Solid Edge part; units mm, degrees
sketch "Sketch1" plane through (0, 0, 0) normal (0, -1, 0) x (1, 0, 0)
  line L0 (25, 129.6172) -> (42.2199, 3)
  line L1 (50, 3) -> (42.2199, 3)
  line L2 (50, 0) -> (50, 3)
  line L3 (50, 0) -> (70, 0)
  line L4 (70, 0) -> (70, 20)
  line L5 (70, 20) -> (50, 20)
  line L6 (33, 145) -> (50, 20)
  line L7 (35, 145) -> (33, 145)
  line L8 (35, 185) -> (35, 145)
  line L9 (25, 185) -> (35, 185)
  line L10 (25, 185) -> (25, 129.6172)
  dimension "D1" = 70
  dimension "D2" = 50
  dimension "D3" = 70
  dimension "D4" = 35
  dimension "D5" = 35
revolve "RevolvedProtrusion1" add sketch "Sketch1" angle 360 about axis through (0, 0, 54) along (0, 0, -1)
fillet "Round_1" radius 8 1 edges at (-50, 0, 20)
fillet "Round_1" radius 1 2 edges at (-50, 0, 3) (-33, 0, 145)
Source: CAD feature listing. Evaluate the final solid. Frame: model axes, mm. A direction names the side the tool comes from. Round coordinates to 2 decimals unless told otherwise and drop trailing zeros. Loops run counter-clockwise (first coordinate to the right, second up) from the corner with the lowest first, then second, coordinate; pieces in that order, holes last.
Q1. Mould query, pull axis Y, two halves, no side actions, for faces 1 (the face through (-48, -17, 0)), 2 (the face through (39.314, -12.381, 84.575)), 3 (the face through (47.69, 15.02, 1.01)). Classes: pulls with the +Y half, pulls with the -Y half, needs draft (parallel to the pull), parting line crosses it, or undercut.
Q2. Access query for faces 4 (the face through (-57.4, -0.3, 20)), 5 (the face through (7.6, 33.5, 145)), 6 (the face through (22, -37, 3)), 7 (the face through (23.846, -7.509, 156.921)). Directions: +Z, -Z, +X, -X, +Y, -Y. A direction counts if a zero-diameter tool reaches every point of the face in a straight line with its end or side. Return the directions, or none.
Q3. Section A-A, the plane x = 0. Return loops of the section in (y, z).
Q4. Ray query, line 1 (X direction, y = 0, z = 0.8); line 2 (X direction, y = 0, z = 172). Return the intervals inside material, ascending.
Q5. Section C-C, the plane z = 17. Return loops of the section in (x, y).
Q6. First-contact query: P1, Ø6, axis at x = -9, z = 132.5, coming from the +Y side; P2, Ø4, axis at y = -23.5, z = 151, coming from the +X side; P3, Ø5, axis at x = 14, z = 161.5, coming from the +Y side. Flat tips, straight axial feed; report the tip coordinate or a pass-through.
Q7. Section D-D, the plane y = 61.5. Return loops of the section in (x, z), plus the area to 3 significant figures.
Solutions:
1. face 1: needs draft
1. face 2: parting line crosses it
1. face 3: undercut
2. face 4: +Z
2. face 5: none
2. face 6: -Z
2. face 7: +Z, -Z
3. outline: (-70, 0) - (-50, 0) - (-50, 2) arc R1 cw to (-49, 3) - (-42.22, 3) - (-25, 129.62) - (-25, 185) - (-35, 185) - (-35, 145) - (-34.15, 145) arc R1 cw to (-33.15, 143.87) - (-49.06, 26.92) arc R8 cw to (-56.99, 20) - (-70, 20) - close; (25, 129.62) - (42.22, 3) - (49, 3) arc R1 cw to (50, 2) - (50, 0) - (70, 0) - (70, 20) - (56.99, 20) arc R8 cw to (49.06, 26.92) - (33.15, 143.87) arc R1 cw to (34.15, 145) - (35, 145) - (35, 185) - (25, 185) - close
4. line 1: x = -70 to -50, 50 to 70
4. line 2: x = -35 to -25, 25 to 35
5. outline: circle Ø140 at (0, 0); hole circle Ø80.63 at (0, 0)
6. P1: stops at y = 34.32
6. P2: stops at x = 27.62
6. P3: stops at y = 33.06
7. outline: (-33.43, 0) - (33.43, 0) - (33.43, 20) - (-33.43, 20) - close
7. area: 1,340 mm2
